Build history of the part. All positions in model axes, mm. A direction names the side the tool comes from. Give positions to 0.01 mm unless a question says otherwise; leave off trailing zeros. Loops run counter-clockwise (first coordinate to the right, second up) from the corner with the lowest first, then second, coordinate; pieces in that order, holes last. Notation, with made-up numbers: M -1.5,-20 L 53.5,-20 A27 cw 53.5,1 Z; hole C -4,21 d6. An arc over 180 degrees is marked long. Answer in a Markdown table with one row per item. Add a question column.
```python
from build123d import *

# Parameters (mm, degrees)
EXTRUDE_1_DEPTH     = 32
SKETCH_2_R          = 3
EXTRUDE_2_DEPTH     = 1.5
SKETCH_3_R          = 1
CUT_EXTRUDE_1_DEPTH = 1.5
SKETCH_4_R          = 1
EXTRUDE_3_DEPTH     = 7


with BuildPart() as part:
    # 草图1 → 凸台-拉伸1 (new body)
    with BuildSketch(Plane(origin=(0, 0, 0), x_dir=(1, 0, 0), z_dir=(0, 1, 0))):
        with BuildLine():
            Line((-10, 7.65), (10, 7.65))
            ThreePointArc((10, 7.65), (13.31807086, 0), (10, -7.65))
            Line((10, -7.65), (-10, -7.65))
            ThreePointArc((-10, -7.65), (-13.31807086, 0), (-10, 7.65))
        make_face()
    extrude(amount=EXTRUDE_1_DEPTH)

    # 草图2 → 凸台-拉伸2 (add)
    with BuildSketch(Plane(origin=(0, 32, 0), x_dir=(1, 0, 0), z_dir=(0, 1, 0))):
        with Locations(Location((0, 0, 0), (0, 0, 270))):
            Circle(SKETCH_2_R)
    extrude(amount=EXTRUDE_2_DEPTH)

    # 草图3 → 切除-拉伸1 (cut)
    with BuildSketch(Plane(origin=(0, 32, 0), x_dir=(1, 0, 0), z_dir=(0, 1, 0))):
        with Locations(Location((-6, 0, 0), (0, 0, 270))):
            Circle(SKETCH_3_R)
        with Locations(Location((6, 0, 0), (0, 0, 270))):
            Circle(SKETCH_3_R)
    extrude(amount=-CUT_EXTRUDE_1_DEPTH, mode=Mode.SUBTRACT)

    # 草图4 → 凸台-拉伸3 (add)
    with BuildSketch(Plane(origin=(0, 33.5, 0), x_dir=(1, 0, 0), z_dir=(0, 1, 0))):
        with Locations(Location((0, 0, 0), (0, 0, 270))):
            Circle(SKETCH_4_R)
    extrude(amount=EXTRUDE_3_DEPTH)


solid = part.part
```
(1) Wall check: line 1 (X direction, y = 31.3, z = 0); line 2 (Y direction, x = 9, z = -5); line 3 (X direction, y = 8.5, z = 0). Give the ranges that are in metal, low to high.
(2) Slice it at D-D, the plane x = 6. Give the cut face in (y, z), then the cut area to 3 significant figures.
(3) Pull direction X, two halves, no side cores. Call faces 1 (the cylindrical face through (-13.317, 15.776, 0.12)), 2 (the flat face through (6, 30.5, 0)), 3 (the cylindrical face through (0.9, 32.74, 2.86)), 4 (the flat face through (1, 33.5, -1)): +X half, -X half, draft (parallel to the pull), parting line (faces both ways), or undercut.
(4) Pin check, flat tips, straight feed: pin 1 (4 mm diameter, centred on x = 2, z = 3.5, fed in from +Y); pin 2 (4 mm diameter, centred on y = 15, z = -5, fed in from -X); pin 3 (5 mm diameter, centred on y = 27.5, z = -6, fed in from -X). Stop position of each tip, or through.
(5) Slice it at A-A, the plane x = 0. Give the cut face in (y, z), then the cut area to 3 significant figures.
(6) Slice it at C-C, the plane y = 5. Give the cut face in (x, z).
(7) Slice it at B-B, the plane z = 0. Give the cut face in (x, y), then the cut area to 3 significant figures.
(8) Tool access for faces 5 (the flat face through (0, 0, 0)), 6 (the cylindrical face through (7, 31, 0)): list every direction of +Z, -Z, +X, -X, +Y, -Y with a clear straight run to the whole face (end or side of a thin tool).
Solution:
| question | item | result |
|---|---|---|
| 1 | line 1 | -13.32 to -7, -5 to 5, 7 to 13.32 |
| 1 | line 2 | 0 to 32 |
| 1 | line 3 | -13.32 to 13.32 |
| 2 | outline | M 0,-7.65 L 32,-7.65 L 32,-1 L 30.5,-1 L 30.5,1 L 32,1 L 32,7.65 L 0,7.65 Z |
| 2 | area | 487 mm^2 |
| 3 | face 1 | -X half |
| 3 | face 2 | undercut |
| 3 | face 3 | parting line |
| 3 | face 4 | draft |
| 4 | pin 1 | y = 33.5 |
| 4 | pin 2 | x = -12.88 |
| 4 | pin 3 | x = -12.72 |
| 5 | outline | M 0,-7.65 L 32,-7.65 L 32,-3 L 33.5,-3 L 33.5,-1 L 40.5,-1 L 40.5,1 L 33.5,1 L 33.5,3 L 32,3 L 32,7.65 L 0,7.65 Z |
| 5 | area | 513 mm^2 |
| 6 | outline | M -10,-7.65 L 10,-7.65 A10.48 ccw 10,7.65 L -10,7.65 A10.48 ccw Z |
| 7 | outline | M -13.32,0 L 13.32,0 L 13.32,32 L 7,32 L 7,30.5 L 5,30.5 L 5,32 L 3,32 L 3,33.5 L 1,33.5 L 1,40.5 L -1,40.5 L -1,33.5 L -3,33.5 L -3,32 L -5,32 L -5,30.5 L -7,30.5 L -7,32 L -13.32,32 Z |
| 7 | area | 869 mm^2 |
| 8 | face 5 | +Z, -Z, +X, -X, -Y |
| 8 | face 6 | +Y |
